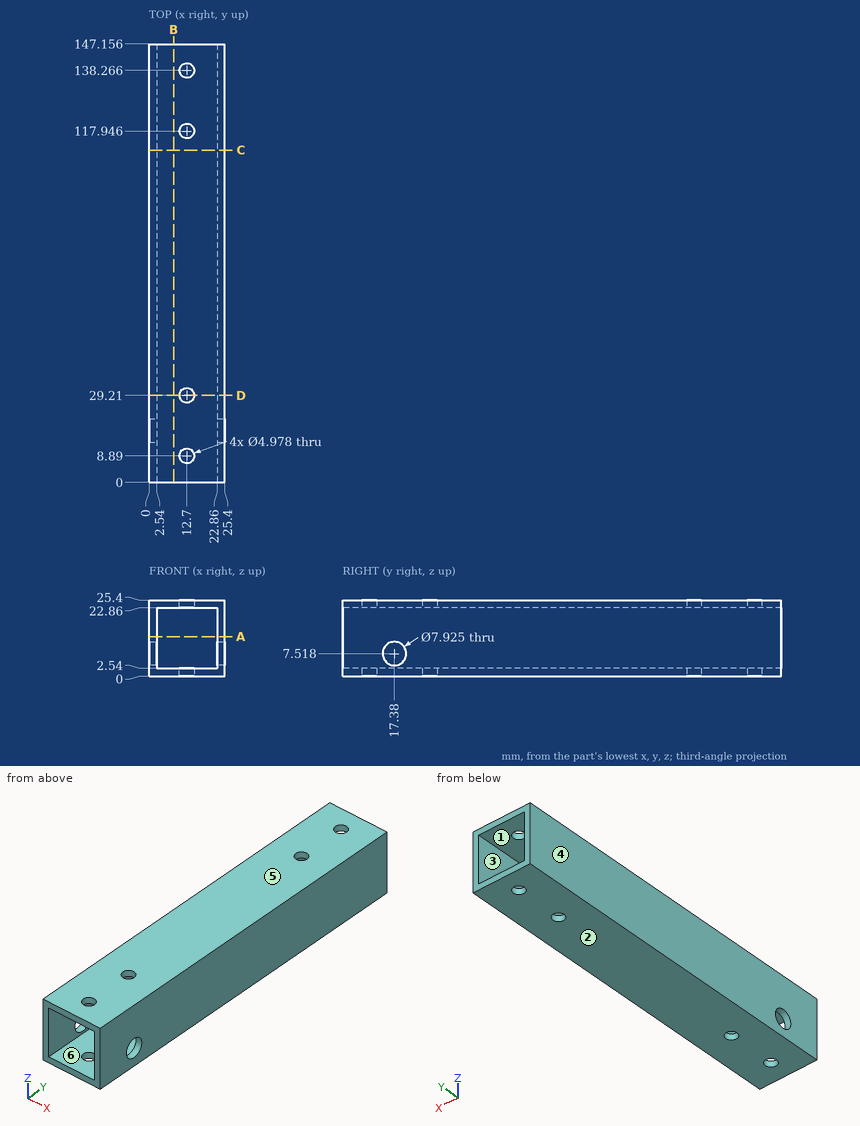
Input: dimensioned drawing with shaded views. Units: mm. Origin: part minimum x, y, z. A direction names the side the tool comes from. Coordinates: 2 decimals unless noted, no trailing zeros. Write each loop counter-clockwise with the first axis right and the second up, starting at its lowest first coordinate (ties: lowest second). Pieces come first, ordered by that corner, then holes. Notation, with made-up numbers: (11, -18) -> (55, -18) arc R18 cw to (55, -10) -> close; hole circle Ø8 at (50.5, 68). An arc over 180 degrees is marked (long way). Return JSON: item names as keys, results as strings. Group by question number.
1) Section query B-B, the plane x = 8.25. Return loops of the section in (y, z) (1 decimal).
2) Ray query, line 1 along Y through (x, z) = (12.7, 24.45) (1 decimal); line 2 along X through (y, z) = (109, 6.5). Return the intervals inside material, ascending.
3) Section query D-D, the plane y = 29.21. Return loops of the section in (x, z), plus the area to 3 significant figures.
4) Section query A-A, the plane z = 13.25. Return loops of the section in (x, y) (1 decimal).
5) Mould query, pull axis X, two halves, no side actions, for the marked faces 3, 4, 5 and 6. Classes: +X half, -X half, draft (parallel to the pull), parting line (faces both ways), or undercut.
6) Section query C-C, the plane y = 111.5. Return loops of the section in (x, z), plus the area to 3 significant figures.
7) Contact query for flat-ended pins moving along their axis: P1, Ø4, axis at x = 12.7, y = 138.27, coming from the -Z side; P2, Ø8, axis at x = 12.7, y = 117.95, coming from the -Z side. Output: stop coordinate, or through.
8) Set-up query: the marked faces 1 and 2. Return all of +Z, -Z, +X, -X, +Y, -Y with unobstructed straight access to the full face (end or side cutting, diameter ignored); none if empty.
From the geometry:
{
 "1": {"outline": "(0, 0) -> (147.2, 0) -> (147.2, 2.5) -> (0, 2.5) -> close; (0, 22.9) -> (147.2, 22.9) -> (147.2, 25.4) -> (0, 25.4) -> close"},
 "2": {"line 1": "0 to 6.4, 11.4 to 26.7, 31.7 to 115.5, 120.4 to 135.8, 140.8 to 147.2", "line 2": "0 to 2.54, 22.86 to 25.4"},
 "3": {"outline": "(0, 0) -> (10.21, 0) -> (10.21, 2.54) -> (2.54, 2.54) -> (2.54, 22.86) -> (10.21, 22.86) -> (10.21, 25.4) -> (0, 25.4) -> close; (15.19, 0) -> (25.4, 0) -> (25.4, 25.4) -> (15.19, 25.4) -> (15.19, 22.86) -> (22.86, 22.86) -> (22.86, 2.54) -> (15.19, 2.54) -> close", "area": "207 mm²"},
 "4": {"outline": "(0, 0) -> (2.5, 0) -> (2.5, 147.2) -> (0, 147.2) -> close; (22.9, 0) -> (25.4, 0) -> (25.4, 147.2) -> (22.9, 147.2) -> close"},
 "5": {"face 3": "undercut", "face 4": "-X half", "face 5": "draft", "face 6": "undercut"},
 "6": {"outline": "(0, 0) -> (25.4, 0) -> (25.4, 25.4) -> (0, 25.4) -> close; hole (2.54, 2.54) -> (22.86, 2.54) -> (22.86, 22.86) -> (2.54, 22.86) -> close", "area": "232 mm²"},
 "7": {"P1": "through", "P2": "z = 0"},
 "8": {"face 1": "+Y, -Y", "face 2": "-Z, +X, -X, +Y, -Y"}
}
